Autodesk Inventor part; units mm, degrees
ref_plane "YZ Plane" through (0, 0, 0) normal (1, 0, 0) x (0, 1, 0)
ref_plane "XZ Plane" through (0, 0, 0) normal (0, 1, 0) x (-1, 0, 0)
ref_plane "XY Plane" through (0, 0, 0) normal (0, 0, 1) x (1, 0, 0)
sketch "Sketch1" plane through (0, 0, 0) normal (0, 0, 1) x (1, 0, 0)
  line L0 (-25, 35) -> (25, 35)
  line L1 (25, 35) -> (25, -35)
  line L2 (25, -35) -> (-25, -35)
  line L3 (-25, -35) -> (-25, 35)
  line L4 (-25, 35) -> (25, -35) construction
  line L5 (25, 35) -> (-25, -35) construction
  circle A0 centre (-20, 30) radius 1.6
  line L6 (0, 0) -> (0, 8.6163)
  line L7 (0, 0) -> (6.049, 0)
  circle A1 centre (20, 30) radius 1.6
  circle A2 centre (-20, -30) radius 1.6
  circle A3 centre (20, -30) radius 1.6
  dimension "d0" = 50
  dimension "d1" = 70
  dimension "d12" = 3.2
  dimension "d13" = 5
  dimension "d18" = 5
extrude "Plate1" add sketch "Sketch1" along normal blind 1
sketch "Sketch2" plane through (0, 0, 1) normal (0, 0, 1) x (1, 0, 0)
  circle A0 centre (-4, 4) radius 1.6
  line L0 (-25, 35) -> (25, 35)
  line L1 (0, 0) -> (10.5452, 0)
  line L2 (-4, 4) -> (-0.3431, 4)
  line L3 (-0.3431, 4) -> (-0.3431, 2.4)
  circle A1 centre (4, 4) radius 1.6
  circle A2 centre (-4, -4) radius 1.6
  circle A3 centre (4, -4) radius 1.6
  point P0 (0, 35)
  dimension "d20" = 3.2
  dimension "d24" = 8
  dimension "d27" = 8
  dimension "d30" = 4
  dimension "d31" = 4
extrude "Extrusion1" cut sketch "Sketch2" against normal blind 10
equation "\"d2\" = 厚度"
equation "\"折彎半徑\" = 厚度"
equation "\"折彎離隙寬度\" = 厚度"
equation "\"折彎離隙深度\" = 0.5 * 厚度"
equation "\"轉角離隙大小\" = 4 * 厚度"
equation "\"最小剩餘\" = 2 * 厚度"
equation "\"轉移半徑\" = 折彎半徑"
equation "\"Jacobi半徑大小\" = 折彎半徑"
equation "\"間隙大小\" = 厚度"
properties part number "signal_combiner_plate"
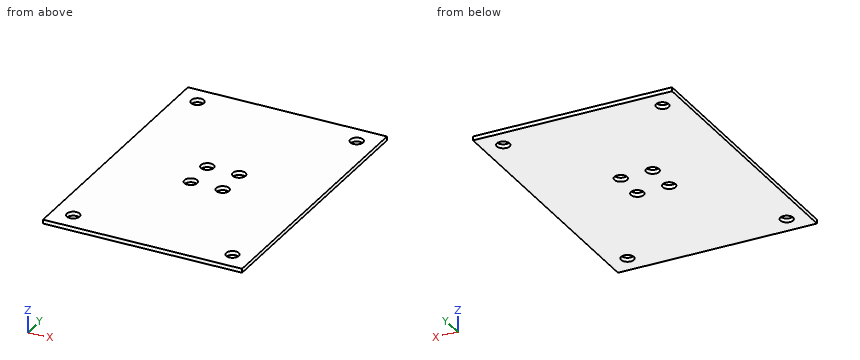
Work out the finished part from the listing and answer in its coordinate system (mm). Coordinates: 2 decimals unless noted, no trailing zeros. Loops run counter-clockwise (first coordinate to the right, second up) from the corner with the lowest first, then second, coordinate; pieces in that order, holes last. Notation, with made-up numbers: M 79,89 L 127,89 A14 ccw 127,108 Z; hole C 19,64.25 d1. An arc over 180 degrees is marked long. Answer in a Markdown table with one row per item. Add a question column.
1. Consider L1, parallel to Y at x = -4, z = 0.7; L2, parallel to Y at x = -20, z = 0.45; L3, parallel to X at y = 5, z = 0.3. Determine where each line is inside the solid, lowest interval first.
2. Find section A-A, the plane y = -4. Write down the section's boundary in (x, z).
3. Find section B-B, the plane x = 20. Write down the section's boundary in (y, z), then the cut area to 3 significant figures.
4. Find section C-C, the plane z = 0.35. State how many separate pieces and enclosed holes the cut face has, then the cut area to 3 significant figures.
Reported:
| question | item | result |
|---|---|---|
| 1 | L1 | y = -35 to -5.6, -2.4 to 2.4, 5.6 to 35 |
| 1 | L2 | y = -35 to -31.6, -28.4 to 28.4, 31.6 to 35 |
| 1 | L3 | x = -25 to -5.25, -2.75 to 2.75, 5.25 to 25 |
| 2 | outline | M -25,0 L -5.6,0 L -5.6,1 L -25,1 Z; M -2.4,0 L 2.4,0 L 2.4,1 L -2.4,1 Z; M 5.6,0 L 25,0 L 25,1 L 5.6,1 Z |
| 3 | outline | M -35,0 L -31.6,0 L -31.6,1 L -35,1 Z; M -28.4,0 L 28.4,0 L 28.4,1 L -28.4,1 Z; M 31.6,0 L 35,0 L 35,1 L 31.6,1 Z |
| 3 | area | 63.6 mm^2 |
| 4 | separate pieces | 1 |
| 4 | enclosed holes | 8 |
| 4 | area | 3,440 mm^2 |
